from build123d import *

# Parameters (mm, degrees)
SKETCH1_R                = 2.5000000000000004
BOSS_EXTRUDE1_DEPTH      = 2
FILLET1_R                = 10
FILLET2_R                = 10
FILLET5_R                = 2
FILLET6_R                = 2
BOSS_EXTRUDE2_DEPTH      = 5.3
BOSS_EXTRUDE2_DEPTH_BACK = 4.5


with BuildPart() as part:
    # Sketch1 → Boss-Extrude1 (new body)
    with BuildSketch(Plane(origin=(0, 0, 0), x_dir=(1, 0, 0), z_dir=(0, 1, 0))):
        with BuildLine():
            Line((4.734439187943633, 4.337505524576787), (-11.123424173439652, -8.60036927980545))
            Line((-11.123424173439652, -8.60036927980545), (-1.3192163601402593, -8.60036927980545))
            Line((-1.3192163601402593, -8.60036927980545), (10.29708605182919, 1.0617245936219641))
            Line((10.29708605182919, 1.0617245936219641), (13.693514413313048, 10.480195617492226))
            ThreePointArc((13.693514413313048, 10.480195617492226), (12.643820805599, 18.747230765158918), (7.611903426882685, 12.104525420451473))
            Line((7.611903426882685, 12.104525420451473), (4.734439187943633, 4.337505524576787))
        make_face()
        with Locations(Location((11.482625796556237, 14.39963072019455, 0), (0, 0, 270))):
            Circle(SKETCH1_R, mode=Mode.SUBTRACT)
    extrude(amount=BOSS_EXTRUDE1_DEPTH)

    # Fillet1
    fillet1_edges = [part.edges().sort_by_distance(p)[0] for p in [
        (10.29708605182919, 1, -1.0617245936219641),
    ]]
    fillet(fillet1_edges, radius=FILLET1_R)

    # Fillet2
    fillet2_edges = [part.edges().sort_by_distance(p)[0] for p in [
        (4.734439187943633, 1, -4.337505524576787),
    ]]
    fillet(fillet2_edges, radius=FILLET2_R)

    # Fillet5
    fillet5_edges = [part.edges().sort_by_distance(p)[0] for p in [
        (6.6461096923169105, 2, -9.49759844281185),
        (4.438286722207531, 2, -4.549211293465088),
        (12.456410034317898, 2, -7.049641368446211),
        (9.999920903343424, 2, -1.270100820961935),
        (-4.249333346620522, 2, 2.9920395518602865),
        (3.4439024153195033, 2, 4.638549149214148),
    ]]
    fillet(fillet5_edges, radius=FILLET5_R - 0.0001)  # a hair under: the kernel refuses the full size

    # Fillet6
    fillet6_edges = [part.edges().sort_by_distance(p)[0] for p in [
        (12.744313913733471, 2, -18.719137994754206),
    ]]
    fillet(fillet6_edges, radius=FILLET6_R - 0.0001)  # a hair under: the kernel refuses the full size

    # Sketch6 → Boss-Extrude2 (add, two sides: drawn at the far end of the back side and taken through both)
    with BuildSketch(Plane(origin=(-6.6499999999999995, 0, 0), x_dir=(0, 0, -1), z_dir=(1, 0, 0)).offset(-BOSS_EXTRUDE2_DEPTH_BACK)):
        Polygon((-8.60036927980545, 2.7250000000000005), (-6.60036927980545, 2), (-6.60036927980545, 0), (-8.60036927980545, -0.7249999999999998), align=None)
    extrude(amount=BOSS_EXTRUDE2_DEPTH + BOSS_EXTRUDE2_DEPTH_BACK)


solid = part.part
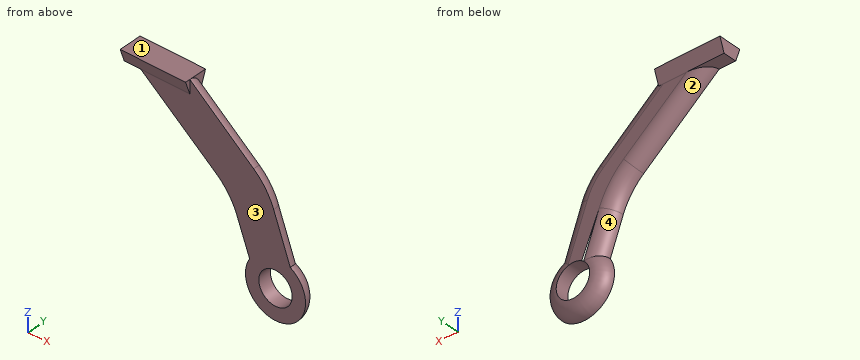
Input: part model. Units: mm. Frame: model coordinates. Face numbers are marked on the shaded views. Coordinates: 2 decimals unless noted, no trailing zeros. Loops run counter-clockwise (first coordinate to the right, second up) from the corner with the lowest first, then second, coordinate; pieces in that order, holes last.
Q1. Cut plane B-B (x = -9). Output: boundary loops of the cut face in (y, z) (3 decimals).
Q2. Draft query along Z for the marked faces 1, 2, 3 and 4. Return one class per face: +Z half, -Z half, draft (parallel to the pull), parting line (faces both ways), or undercut.
Q3. Contact query for flat-ended pins moving along their axis: pin 1 (12.5 mm diameter, centred on x = 7, z = 0.5, fed in from -Y); pin 2 (1.6 mm diameter, centred on x = -8.5, y = 1.5, fed in from -Z); pin 3 (0.6 mm diameter, centred on y = -0.5, z = 8, fed in from +X); pin 4 (5 mm diameter, centred on x = 10, z = 3, fed in from +Y). Output: stop coordinate, or through.
Q4. Cut plane A-A (y = 1.35). Output: boundary loops of the cut face in (x, z), then the cut area to 3 significant figures.
Q5. Material intervals for line 1 (Z direction, x = -8, y = 1.25); line 2 (Y direction, x = 8.25, z = -2.5); line 3 (X direction, y = 0.8, z = -17), sorted ascending.
Working result:
1. outline: (-0.725, 8.6) - (0, 6.6) - (2, 6.6) - (2.725, 8.6) - close
2. face 1: +Z half
2. face 2: -Z half
2. face 3: draft
2. face 4: undercut
3. pin 1: stops at y = 0
3. pin 2: stops at z = 6.29
3. pin 3: stops at x = -1.35
3. pin 4: passes through
4. outline: (-11.15, 6.6) - (-7.84, 6.6) - (2.96, -2.21) arc R10.52 cw to (6.17, -6.71) - (8.19, -12.17) arc R3.98 ccw (long way) to (13.27, -10.85) - (10.73, -3.8) arc R9.48 ccw to (7.87, 0.27) - (-1.35, 7.94) - (-1.35, 8.6) - (-11.15, 8.6) - close; hole circle Ø5 at (11.48, -14.4)
4. area: 171 mm2
5. line 1: z = 6.6 to 8.6
5. line 2: y = 0 to 2
5. line 3: x = 8.02 to 14.95
